```python
from build123d import *

# Parameters (mm, degrees)
SKETCH2_W           = 99
SKETCH2_H           = 61
SKETCH2_W_2         = 89.5
SKETCH2_H_2         = 42
BOSS_EXTRUDE1_DEPTH = 1.6
SKETCH3_R           = 1.375
BOSS_EXTRUDE2_DEPTH = 2.4


with BuildPart() as part:
    # Sketch2 → Boss-Extrude1 (new body)
    with BuildSketch(Plane.XY):
        with Locations((49.5, 30.5)):
            Rectangle(SKETCH2_W, SKETCH2_H)
        with Locations((49.5, 30.5)):
            Rectangle(SKETCH2_W_2, SKETCH2_H_2, mode=Mode.SUBTRACT)
    extrude(amount=-BOSS_EXTRUDE1_DEPTH)

    # Sketch3 → Boss-Extrude2 (add)
    with BuildSketch(Plane.XY):
        with Locations(Location((3, 58, 0), (0, 0, 180))):
            Circle(SKETCH3_R)
        with Locations(Location((96, 58, 0), (0, 0, 180))):
            Circle(SKETCH3_R)
        with Locations(Location((96, 3, 0), (0, 0, 180))):
            Circle(SKETCH3_R)
        with Locations(Location((3, 3, 0), (0, 0, 180))):
            Circle(SKETCH3_R)
    extrude(amount=BOSS_EXTRUDE2_DEPTH)


solid = part.part
```
Could you check a few things on this model? Use its own coordinates, in mm. A direction names the side the tool comes from. Give positions to 0.01 mm unless a question says otherwise; leave off trailing zeros. Order: outer loops, then holes, each group sorted by start corner. A loop starts at its lowest first (then second) coordinate and runs counter-clockwise, first axis right, second up.
Q1. We'd pull the mould along Y, two halves only. Please class faces 1 (the cylindrical face through (3.3, 59.34, 1.18)), 2 (the flat face through (96, 58, 2.4)): +Y half, -Y half, draft (parallel to the pull), parting line (faces both ways), or undercut.
Q2. If I drill on line 1 along Y through (x, z) = (12.5, -1.2); line 2 along X through (y, z) = (44, -0.5); line 3 along Z through (x, y) = (4.5, 16), over which ranges is the centre line in solid material (lowest first)?
Q3. I'm going to push a flat-ended pin straight in: P1, Ø2, axis at y = 51.5, z = 1.5, coming from the +X side. Where does the tip first touch, or does it pass through?
Q4. Suppose I cut it at B-B, the plane x = 91.5. Write out the boundary of the cut face in (y, z), and give its area (3 significant figures).
Q5. For faces 3 (the cylindrical face through (2.37, 4.22, 1.18)), 4 (the flat face through (49, 53, -1.6)), which set-ups out of +Z, -Z, +X, -X, +Y, -Y let a thin tool reach every point of the face, with its end or its side?
Q6. Suppose I cut it at C-C, the plane z = 1.15. Write out the boundary of the cut face in (x, y) (3 decimals), and give its area (3 significant figures).
Q7. Suppose I cut it at D-D, the plane y = 58. Write out the boundary of the cut face in (x, z) (3 decimals), and give its area (3 significant figures).
Q8. Suppose I cut it at A-A, the plane y = 25. Write out the boundary of the cut face in (x, z), and give its area (3 significant figures).
Solution:
1. face 1: undercut
1. face 2: draft
2. line 1: y = 0 to 9.5, 51.5 to 61
2. line 2: x = 0 to 4.75, 94.25 to 99
2. line 3: z = -1.6 to 0
3. P1: passes through
4. outline: (0, -1.6) - (9.5, -1.6) - (9.5, 0) - (0, 0) - close; (51.5, -1.6) - (61, -1.6) - (61, 0) - (51.5, 0) - close
4. area: 30.4 mm2
5. face 3: +Z
5. face 4: -Z, +X, -X, +Y, -Y
6. outline: circle Ø2.75 at (3, 3); circle Ø2.75 at (3, 58); circle Ø2.75 at (96, 3); circle Ø2.75 at (96, 58)
6. area: 23.8 mm2
7. outline: (0, -1.6) - (99, -1.6) - (99, 0) - (97.375, 0) - (97.375, 2.4) - (94.625, 2.4) - (94.625, 0) - (4.375, 0) - (4.375, 2.4) - (1.625, 2.4) - (1.625, 0) - (0, 0) - close
7. area: 172 mm2
8. outline: (0, -1.6) - (4.75, -1.6) - (4.75, 0) - (0, 0) - close; (94.25, -1.6) - (99, -1.6) - (99, 0) - (94.25, 0) - close
8. area: 15.2 mm2
